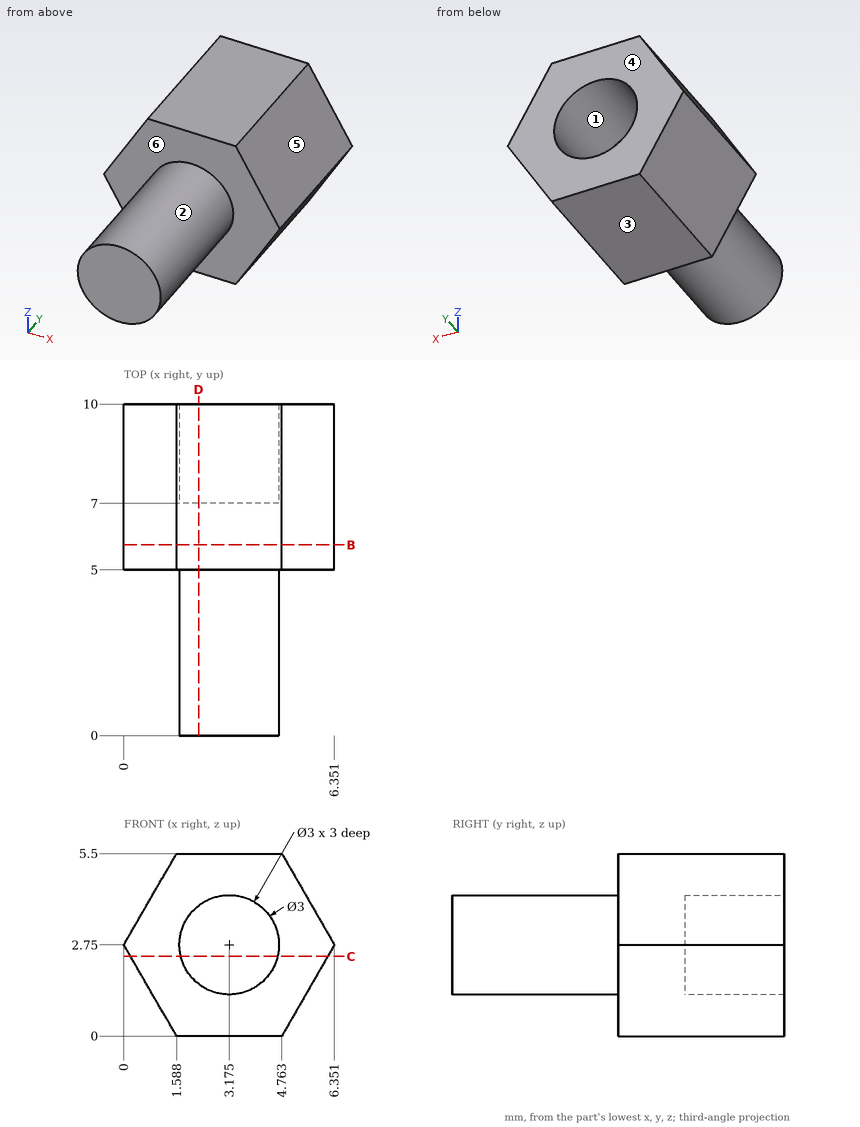
The figure shows three views and two pictorial views of one solid part (mm, origin at its lowest corner). Answer the questions. A direction names the side the tool comes from. Round coordinates to 2 decimals unless told otherwise and drop trailing zeros. Order: outer loops, then holes, each group sorted by start corner. A loop starts at its lowest first (then second) coordinate and runs counter-clockwise, first axis right, second up. Notation, with made-up numbers: (-32, 42.25) - (22, 42.25) arc R19 cw to (22, 67.25) - close; hole circle Ø2 at (27, -17). An arc over 180 degrees is marked (long way). Write item = value, one per line. Start each with the question number.
1) Given pin 1 (2 mm diameter, centred on y = 6.5, z = 5, fed in from -X), flat-ended and moving along its own axis, determine where the tip first touches the part or whether it passes through.
2) Section C-C, the plane z = 2.4 is taken. Write down the section's boundary in (x, y).
3) For a pull along Z with two mould halves and no side action, classify the marked faces 1, 2, 3 and 4 as released by +Z, released by -Z, zero draft, split by the parting line, or undercut.
4) Section B-B, the plane y = 5.75 is taken. Write down the section's boundary in (x, z), plus the area to 3 significant figures.
5) Straight lines are drawn through the part: L1, parallel to Y at x = 1.75, z = 4.45; L2, parallel to Z at x = 2.75, y = 9; L3, parallel to Z at x = 2, y = 7.25. For each, find the intervals that lie inside material, in ascending order.
6) Section D-D, the plane x = 2.25 is taken. Write down the section's boundary in (y, z).
7) For the marked faces 5 and 6, determine the directions among +Z, -Z, +X, -X, +Y, -Y from which every point of the face is accessible in a straight line to the end or side of a thin tool.
Results list:
q1.pin_1 = 0.72
q2.outline = (0.2, 5) - (1.72, 5) - (1.72, 0) - (4.63, 0) - (4.63, 5) - (6.15, 5) - (6.15, 10) - (4.63, 10) - (4.63, 7) - (1.72, 7) - (1.72, 10) - (0.2, 10) - close
q3.face_1 = undercut
q3.face_2 = split by the parting line
q3.face_3 = released by -Z
q3.face_4 = zero draft
q4.outline = (0, 2.75) - (1.59, 0) - (4.76, 0) - (6.35, 2.75) - (4.76, 5.5) - (1.59, 5.5) - close
q4.area = 26.2 mm^2
q5.L1 = 5 to 10
q5.L2 = 0 to 1.31, 4.19 to 5.5
q5.L3 = 0 to 1.82, 3.68 to 5.5
q6.outline = (0, 1.57) - (5, 1.57) - (5, 0) - (10, 0) - (10, 1.57) - (7, 1.57) - (7, 3.93) - (10, 3.93) - (10, 5.5) - (5, 5.5) - (5, 3.93) - (0, 3.93) - close
q7.face_5 = +Z, +X, +Y, -Y
q7.face_6 = -Y
